Build history of the part. All positions in model axes, mm. Face numbers are marked on the shaded views. A direction names the side the tool comes from. Round coordinates to 2 decimals unless told otherwise and drop trailing zeros. Write each loop counter-clockwise with the first axis right and the second up, starting at its lowest first coordinate (ties: lowest second). Pieces come first, ordered by that corner, then holes.
Autodesk Inventor part; units mm, degrees
ref_plane "YZ Plane" through (0, 0, 0) normal (1, 0, 0) x (0, 1, 0)
ref_plane "XZ Plane" through (0, 0, 0) normal (0, 1, 0) x (-1, 0, 0)
ref_plane "XY Plane" through (0, 0, 0) normal (0, 0, 1) x (1, 0, 0)
sketch "Sketch1" plane through (0, 0, 0) normal (0, 0, 1) x (1, 0, 0)
  circle A0 centre (0, 0) radius 6.22 construction
  circle A1 centre (0, 0) radius 2.8
  line L0 (-0.675, 0.675) -> (-0.675, 2.025)
  line L1 (-0.675, 2.025) -> (0.675, 2.025)
  line L2 (0.675, 2.025) -> (0.675, 0.675)
  line L3 (0.675, 0.675) -> (2.025, 0.675)
  line L4 (2.025, 0.675) -> (2.025, -0.675)
  line L5 (2.025, -0.675) -> (0.675, -0.675)
  line L6 (0.675, -0.675) -> (0.675, -2.025)
  line L7 (0.675, -2.025) -> (-0.675, -2.025)
  line L8 (-0.675, -2.025) -> (-0.675, -0.675)
  line L9 (-0.675, -0.675) -> (-2.025, -0.675)
  line L10 (-2.025, -0.675) -> (-2.025, 0.675)
  line L11 (-2.025, 0.675) -> (-0.675, 0.675)
  circle A2 centre (0, 0) radius 5.75
  point P0 (-6.07, -6.1)
  dimension "d0" = 12.44
  dimension "d1" = 0.47
extrude "Extrusion1" add sketch "Sketch1" along normal blind 5 contours A1 | L0 L1 L2 L3 L4 L5 L6 L7 L8 L9 L10 L11 | A2
extrude "Extrusion2" add sketch "Sketch1" against normal blind 4.8 contours A1
sketch "Sketch2" plane through (0, 0, 5) normal (0, 0, 1) x (1, 0, 0)
  point P0 (0, 0)
sketch "Sketch3" plane through (0, 0, 5) normal (0, 0, 1) x (1, 0, 0)
  line L0 (-3.7906, 1.642) -> (3.8677, 1.642) construction
  line L1 (3.8677, 1.642) -> (3.8677, -1.5876) construction
  line L2 (3.8677, -1.5876) -> (-3.7906, -1.5876) construction
  line L3 (-3.7906, -1.5876) -> (-3.7906, 1.642) construction
  line L4 (-3.803, -1.4674) -> (-2.7723, 1.5826)
  line L5 (-2.7723, 1.5826) -> (-1.9369, 1.5826)
  line L6 (-1.9369, 1.5826) -> (-0.9062, -1.4674)
  line L7 (-0.9062, -1.4674) -> (-1.6947, -1.4674)
  line L8 (-1.6947, -1.4674) -> (-1.885, -0.8445)
  line L9 (-1.885, -0.8445) -> (-2.844, -0.8445)
  line L10 (-2.844, -0.8445) -> (-3.0368, -1.4674)
  line L11 (-3.0368, -1.4674) -> (-3.803, -1.4674)
  line L12 (-2.0531, -0.2909) -> (-2.3645, 0.7176)
  line L13 (-2.3645, 0.7176) -> (-2.6784, -0.2909)
  line L14 (-2.6784, -0.2909) -> (-2.0531, -0.2909)
  line L15 (0.6633, -0.4046) -> (-0.6937, -0.4046)
  line L16 (-0.6937, -0.4046) -> (-0.6937, 0.1639)
  line L17 (-0.6937, 0.1639) -> (0.6633, 0.1639)
  line L18 (0.6633, 0.1639) -> (0.6633, -0.4046)
  spline S0 degree 2 poles (3.7528, -1.2944) (3.5526, -1.3759) (2.9125, -1.5316) (2.601, -1.5316) knots 0 0 0 1 2 2 2
  spline S1 degree 2 poles (2.601, -1.5316) (1.8818, -1.5316) (1.0291, -0.7012) (1.0291, 0.0601) knots 0 0 0 1 2 2 2
  spline S2 degree 2 poles (1.0291, 0.0601) (1.0291, 0.7769) (1.8818, 1.642) (2.6233, 1.642) knots 0 0 0 1 2 2 2
  spline S3 degree 2 poles (2.6233, 1.642) (3.0064, 1.642) (3.4859, 1.4961) (3.7405, 1.3725) knots 0 0 0 1 2 2 2
  line L19 (3.7405, 1.3725) -> (3.7405, 0.6558)
  line L20 (3.7405, 0.6558) -> (3.6712, 0.6558)
  spline S4 degree 2 poles (3.6712, 0.6558) (3.6169, 0.6978) (3.4093, 0.8584) (3.3104, 0.9128) knots 0 0 0 1 2 2 2
  spline S5 degree 2 poles (3.3104, 0.9128) (3.1967, 0.9796) (2.8952, 1.0735) (2.7271, 1.0735) knots 0 0 0 1 2 2 2
  spline S6 degree 2 poles (2.7271, 1.0735) (2.5318, 1.0735) (2.208, 0.9499) (2.082, 0.8238) knots 0 0 0 1 2 2 2
  spline S7 degree 2 poles (2.082, 0.8238) (1.9609, 0.7003) (1.82, 0.3221) (1.82, 0.0725) knots 0 0 0 1 2 2 2
  spline S8 degree 2 poles (1.82, 0.0725) (1.82, -0.4614) (2.3563, -0.9706) (2.8185, -0.9706) knots 0 0 0 1 2 2 2
  spline S9 degree 2 poles (2.8185, -0.9706) (2.8606, -0.9706) (2.9693, -0.9656) (3.0113, -0.9632) knots 0 0 0 1 2 2 2
  line L21 (3.0113, -0.9632) -> (3.0113, -0.3625)
  line L22 (3.0113, -0.3625) -> (2.4206, -0.3625)
  line L23 (2.4206, -0.3625) -> (2.4206, 0.2084)
  line L24 (2.4206, 0.2084) -> (3.7528, 0.2084)
  line L25 (3.7528, 0.2084) -> (3.7528, -1.2944)
  point P0 (0.0385, -1.5876)
  point P1 (3.8677, 0.0272)
  point P2 (0, 0.1089)
  point P3 (0, 0.1089)
extrude "Extrusion7" add sketch "Sketch3" along normal blind 0.9
properties part number "IPC A-G key"
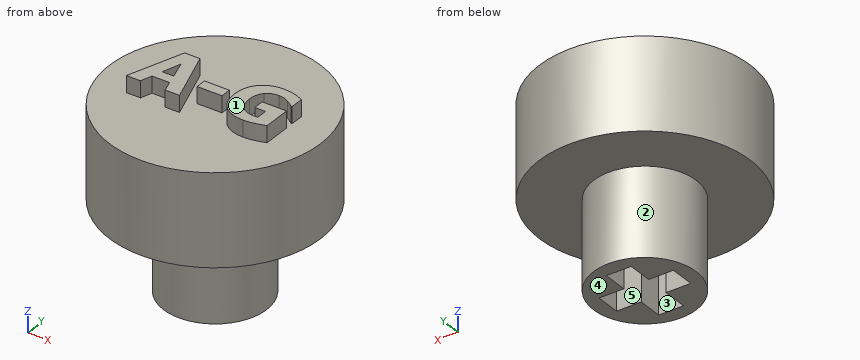
1) Which spindle directions (+Z, -Z, +X, -X, +Y, -Y) get a long thin tool onto all of the face, cutting with end or side? Do the marked faces 4 and 5. Say none if no direction does.
Results:
face 4: -Z, +X, -X, +Y, -Y
face 5: -Z
2) Slice it at B-B (x = 0). Write the cut outline in (y, z) (3 decimals).
Results:
outline: (-5.75, 0) - (-2.8, 0) - (-2.8, -4.8) - (-2.025, -4.8) - (-2.025, 0) - (2.025, 0) - (2.025, -4.8) - (2.8, -4.8) - (2.8, 0) - (5.75, 0) - (5.75, 5) - (0.164, 5) - (0.164, 5.9) - (-0.405, 5.9) - (-0.405, 5) - (-5.75, 5) - close
3) Slice it at A-A (z = -3). Write the cut outline in (x, y) (3 decimals), plus the area to 3 significant figures.
Results:
outline: circle Ø5.6 at (0, 0); hole (-2.025, -0.675) - (-0.675, -0.675) - (-0.675, -2.025) - (0.675, -2.025) - (0.675, -0.675) - (2.025, -0.675) - (2.025, 0.675) - (0.675, 0.675) - (0.675, 2.025) - (-0.675, 2.025) - (-0.675, 0.675) - (-2.025, 0.675) - close
area: 15.5 mm2
4) Slice it at C-C (z = 1.75). Write the cut outline in (x, y).
Results:
outline: circle Ø11.5 at (0, 0)
5) Pin check, flat tips, straight feed: pin 1 Ø1.5 at (x, z) = (1.5, -2.5) entering from -Y; pin 2 Ø3 at (x, z) = (2.5, 1) entering from -Y; pin 3 Ø1.1 at (y, z) = (1.5, -3) entering from +X. Stop position of each tip, or through.
Results:
pin 1: stops at y = -2.7
pin 2: stops at y = -5.66
pin 3: stops at x = 2.63
6) Slice it at D-D (x = -1.25). Write the cut outline in (y, z) (1 decimal).
Results:
outline: (-5.6, 0) - (-2.5, 0) - (-2.5, -4.8) - (-0.7, -4.8) - (-0.7, 0) - (0.7, 0) - (0.7, -4.8) - (2.5, -4.8) - (2.5, 0) - (5.6, 0) - (5.6, 5) - (-0.5, 5) - (-0.5, 5.9) - (-1.5, 5.9) - (-1.5, 5) - (-5.6, 5) - close
7) Mould opens along X. For the marked faces 1, 2 and 3 say: released by +X, released by -X, zero draft, split by the parting line, or undercut.
Results:
face 1: zero draft
face 2: split by the parting line
face 3: undercut
8) Wall check: L1, parallel to Z at x = -4.5, y = 3.5; L2, parallel to Z at x = -1, y = -1.5; L3, parallel to Y at x = -4.75, z = 0.75. Give the ranges that are in metal, low to high.
Results:
L1: z = 0 to 5
L2: z = -4.8 to 5
L3: y = -3.24 to 3.24
